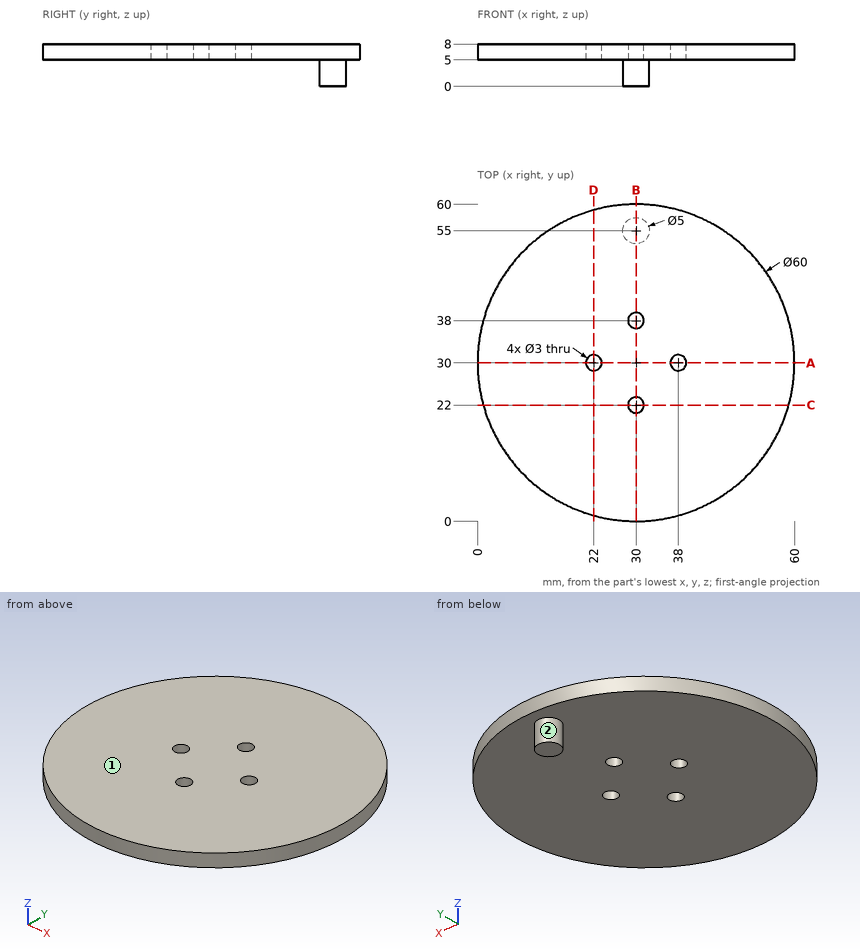
Could you check a few things on this drawing? It's one solid part, dimensions in mm from its lowest x, y, z. A direction names the side the tool comes from. Round coordinates to 2 decimals unless told otherwise and drop trailing zeros. Write each loop counter-clockwise with the first axis right and the second up, starting at its lowest first coordinate (ties: lowest second). Pieces come first, ordered by that corner, then holes.
Q1. If we section it at A-A on y = 30: Write out the boundary of the cut face in (x, z).
Q2. If we section it at B-B on x = 30: Write out the boundary of the cut face in (y, z), plus the area to 3 significant figures.
Q3. Please list where these lines run through material, in increasing order: probe 1 along Z at (x, y) = (4, 22); probe 2 along Y at (x, z) = (38, 6.9); probe 3 along X at (y, z) = (3.5, 6).
Q4. Which directions (+Z, -Z, +X, -X, +Y, -Y) give clear straight access to the entire face, cutting with the end or side of a thin tool? Please do the marked faces 1 and 2.
Q5. Will these pins go through, and if not, where does the flat tip stop? P1, Ø1.5, axis at y = 35, z = 4.5, coming from the +X side; P2, Ø5, axis at x = 46.5, y = 34.5, coming from the -Z side; P3, Ø2.5, axis at x = 22, y = 30, coming from the +Z side; P4, Ø3, axis at x = 8, z = 6, coming from the -Y side.
Q6. If we section it at C-C on y = 22: Write out the boundary of the cut face in (x, z).
Answer below:
1. outline: (0, 5) - (20.5, 5) - (20.5, 8) - (0, 8) - close; (23.5, 5) - (36.5, 5) - (36.5, 8) - (23.5, 8) - close; (39.5, 5) - (60, 5) - (60, 8) - (39.5, 8) - close
2. outline: (0, 5) - (20.5, 5) - (20.5, 8) - (0, 8) - close; (23.5, 5) - (36.5, 5) - (36.5, 8) - (23.5, 8) - close; (39.5, 5) - (52.5, 5) - (52.5, 0) - (57.5, 0) - (57.5, 5) - (60, 5) - (60, 8) - (39.5, 8) - close
2. area: 187 mm2
3. probe 1: z = 5 to 8
3. probe 2: y = 1.09 to 28.5, 31.5 to 58.91
3. probe 3: x = 15.94 to 44.06
4. face 1: +Z, +X, -X, +Y, -Y
4. face 2: -Z
5. P1: stops at x = 59.67
5. P2: stops at z = 5
5. P3: passes through
5. P4: stops at y = 8.1
6. outline: (1.09, 5) - (28.5, 5) - (28.5, 8) - (1.09, 8) - close; (31.5, 5) - (58.91, 5) - (58.91, 8) - (31.5, 8) - close
